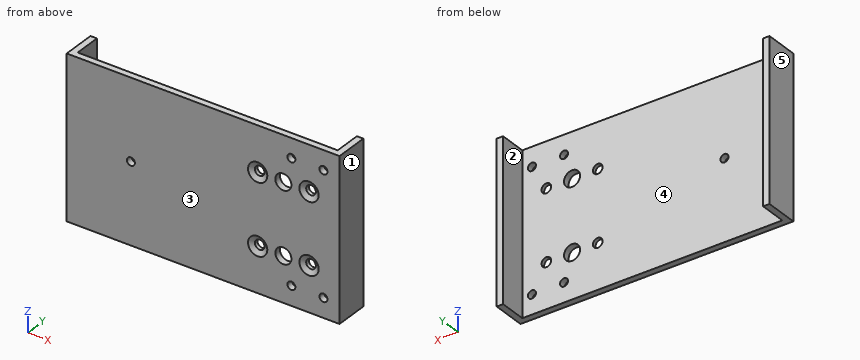
from build123d import *

# Parameters (mm, degrees)
EXTRUDE_1_DEPTH     = 100
SKETCH_2_R          = 5
SKETCH_2_R_2        = 2.5
SKETCH_2_R_3        = 3
CUT_EXTRUDE_1_DEPTH = 4
CHAMFER_3_SIZE      = 3
CHAMFER_3_SIZE2     = 1.732050808
CHAMFER_4_SIZE      = 3
CHAMFER_4_SIZE2     = 1.732050808
CHAMFER_5_SIZE      = 3
CHAMFER_5_SIZE2     = 1.732050808
CHAMFER_6_SIZE      = 3
CHAMFER_6_SIZE2     = 1.732050808


with BuildPart() as part:
    # Эскиз1 → Бобышка-Вытянуть1 (new body)
    with BuildSketch(Plane.XY):
        Polygon((0, 0), (170, 0), (170, 20.7), (166, 20.7), (166, 4), (4, 4), (4, 20.7), (0, 20.7), align=None)
    extrude(amount=EXTRUDE_1_DEPTH)

    # Эскиз2 → Вырез-Вытянуть1 (cut)
    with BuildSketch(Plane.XZ):
        with Locations(Location((135, 72, 0), (0, 0, 270))):
            Circle(SKETCH_2_R)
        with Locations(Location((135, 28, 0), (0, 0, 270))):
            Circle(SKETCH_2_R)
        with Locations(Location((40, 50, 0), (0, 0, 270))):
            Circle(SKETCH_2_R_2)
        with Locations(Location((160, 88, 0), (0, 0, 270))):
            Circle(SKETCH_2_R_2)
        with Locations(Location((140, 88, 0), (0, 0, 270))):
            Circle(SKETCH_2_R_2)
        with Locations(Location((160, 12, 0), (0, 0, 270))):
            Circle(SKETCH_2_R_2)
        with Locations(Location((140, 12, 0), (0, 0, 270))):
            Circle(SKETCH_2_R_2)
        with Locations(Location((151, 28, 0), (0, 0, 270))):
            Circle(SKETCH_2_R_3)
        with Locations(Location((119, 28, 0), (0, 0, 270))):
            Circle(SKETCH_2_R_3)
        with Locations(Location((151, 72, 0), (0, 0, 270))):
            Circle(SKETCH_2_R_3)
        with Locations(Location((119, 72, 0), (0, 0, 270))):
            Circle(SKETCH_2_R_3)
    extrude(amount=-CUT_EXTRUDE_1_DEPTH, mode=Mode.SUBTRACT)

    # Фаска3
    chamfer_3_edges = [part.edges().sort_by_distance(p)[0] for p in [
        (151, 0, 75),
    ]]
    chamfer_3_side = [part.faces().sort_by_distance(p)[0] for p in [
        (83.933938281, 0, 50),
    ]]
    chamfer(chamfer_3_edges, length=CHAMFER_3_SIZE, length2=CHAMFER_3_SIZE2, reference=chamfer_3_side[0])

    # Фаска4
    chamfer_4_edges = [part.edges().sort_by_distance(p)[0] for p in [
        (119, 0, 75),
    ]]
    chamfer_4_side = [part.faces().sort_by_distance(p)[0] for p in [
        (83.590141536, 0, 49.887222715),
    ]]
    chamfer(chamfer_4_edges, length=CHAMFER_4_SIZE, length2=CHAMFER_4_SIZE2, reference=chamfer_4_side[0])

    # Фаска5
    chamfer_5_edges = [part.edges().sort_by_distance(p)[0] for p in [
        (119, 0, 31),
    ]]
    chamfer_5_side = [part.faces().sort_by_distance(p)[0] for p in [
        (83.407686787, 0, 49.773283224),
    ]]
    chamfer(chamfer_5_edges, length=CHAMFER_5_SIZE, length2=CHAMFER_5_SIZE2, reference=chamfer_5_side[0])

    # Фаска6
    chamfer_6_edges = [part.edges().sort_by_distance(p)[0] for p in [
        (151, 0, 31),
    ]]
    chamfer_6_side = [part.faces().sort_by_distance(p)[0] for p in [
        (83.223342048, 0, 49.88605449),
    ]]
    chamfer(chamfer_6_edges, length=CHAMFER_6_SIZE, length2=CHAMFER_6_SIZE2, reference=chamfer_6_side[0])


solid = part.part
Part model, mm, in its own coordinate system. Face numbers are marked on the shaded views. A direction names the side the tool comes from. Coordinates: 2 decimals unless noted, no trailing zeros. Write each loop counter-clockwise with the first axis right and the second up, starting at its lowest first coordinate (ties: lowest second). Pieces come first, ordered by that corner, then holes. Notation, with made-up numbers: (-34.5, 5) - (13.5, 5) arc R26 cw to (13.5, 33) - close; hole circle Ø10 at (0, -31.75). An arc over 180 degrees is marked (long way). Put each result on its own line as item: value.
1. Band-saw the part on B-B (z = 50). Write the cut outline in (x, y).
Final values:
outline: (0, 0) - (37.5, 0) - (37.5, 4) - (4, 4) - (4, 20.7) - (0, 20.7) - close; (42.5, 0) - (170, 0) - (170, 20.7) - (166, 20.7) - (166, 4) - (42.5, 4) - close
2. Probe line 1 along X through (y, z) = (3.3, 72); line 2 along X through (y, z) = (2.4, 88); line 3 along X through (y, z) = (2.1, 50). List the from-to ranges inside material, lowest first. Write a range as [from, to].
Final values:
line 1: x = [0, 116], [122, 130], [140, 148], [154, 170]
line 2: x = [0, 137.5], [142.5, 157.5], [162.5, 170]
line 3: x = [0, 37.5], [42.5, 170]
3. Two-plate mould, pull along X, no slides. Class the marked faces 1, 2 and 3: +X half, -X half, draft (parallel to the pull), parting line (faces both ways), or undercut.
Final values:
face 1: +X half
face 2: undercut
face 3: draft
4. 3-axis set-ups, long thin cutter, end or side, ignore diameter. For the marked faces 4 and 5: which of +Z, -Z, +X, -X, +Y, -Y reach the whole face in a straight line?
Final values:
face 4: +Z, -Z, +Y
face 5: +Z, -Z, -X, +Y, -Y
5. Flat gauge pin, fed straight in: pin 1 Ø3 at (x, z) = (123, 77) entering from +Y. Where does the tip first touch, or does it go through?
Final values:
pin 1: stops at y = 4
6. Band-saw the part on D-D (y = 12). Write the cut outline in (x, z), then the cut area to 3 significant figures.
Final values:
outline: (0, 0) - (4, 0) - (4, 100) - (0, 100) - close; (166, 0) - (170, 0) - (170, 100) - (166, 100) - close
area: 800 mm²
7. Band-saw the part on C-C (x = 40). Write the cut outline in (y, z), then the cut area to 3 significant figures.
Final values:
outline: (0, 0) - (4, 0) - (4, 47.5) - (0, 47.5) - close; (0, 52.5) - (4, 52.5) - (4, 100) - (0, 100) - close
area: 380 mm²
8. Band-saw the part on A-A (x = 135). Write the cut outline in (y, z).
Final values:
outline: (0, 0) - (4, 0) - (4, 23) - (0, 23) - close; (0, 33) - (4, 33) - (4, 67) - (0, 67) - close; (0, 77) - (4, 77) - (4, 100) - (0, 100) - close
